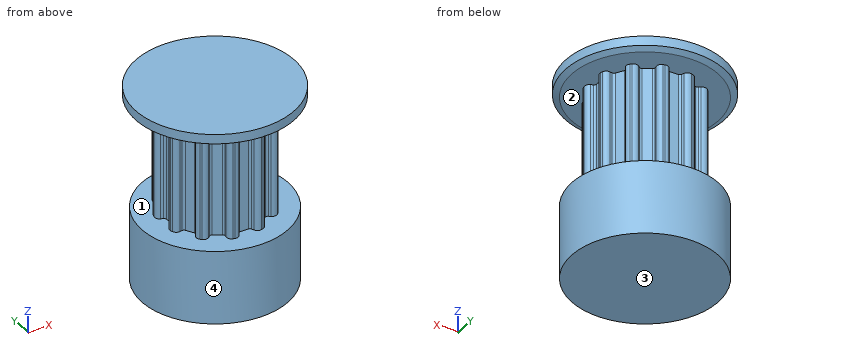
```python
from build123d import *

# Parameters (mm, degrees)
SKETCH5_W           = 10
SKETCH5_H           = 4.5
SKETCH16_W          = 6
SKETCH16_H          = 6
CUT_TOOTH_DEPTH     = 10
PATTERN_TOOTH_COUNT = 12


with BuildPart() as part:
    # Sketch5 → body (revolve)
    with BuildSketch(Plane(origin=(0, 0, 0), x_dir=(0, 0, -1), z_dir=(1, 0, 0))):
        with Locations((5, 2.25)):
            Rectangle(SKETCH5_W, SKETCH5_H)
    revolve(axis=Axis((0, 0, 0), (0, 0, -1)))

    # Sketch16 → body-hub (revolve)
    with BuildSketch(Plane(origin=(0, 0, 0), x_dir=(0, 0, -1), z_dir=(1, 0, 0))):
        with Locations((13, 3)):
            Rectangle(SKETCH16_W, SKETCH16_H)
    revolve(axis=Axis((0, 0, -16), (0, 0, 1)))

    # Sketch23 → cut-tooth (cut)
    with BuildSketch(Plane.XY):
        with BuildLine():
            Line((0.547897017, 3.931595971), (0.6147699, 4.11532771))
            ThreePointArc((0.6147699, 4.11532771), (0.802803604, 4.331669589), (1.087295431, 4.366667911))
            Line((1.087295431, 4.366667911), (1.087295431, 4.933335822))
            Line((1.087295431, 4.933335822), (-1.087295431, 4.933335822))
            Line((-1.087295431, 4.933335822), (-1.087295431, 4.366667911))
            ThreePointArc((-1.087295431, 4.366667911), (-0.802803604, 4.331669589), (-0.6147699, 4.11532771))
            Line((-0.6147699, 4.11532771), (-0.547897017, 3.931595971))
            ThreePointArc((-0.547897017, 3.931595971), (-0.47467378, 3.836169591), (-0.359958492, 3.8))
            Line((-0.359958492, 3.8), (0.359958492, 3.8))
            ThreePointArc((0.359958492, 3.8), (0.47467378, 3.836169591), (0.547897017, 3.931595971))
        make_face()
    cut_tooth = extrude(amount=-CUT_TOOTH_DEPTH, mode=Mode.SUBTRACT)

    # pattern-tooth: cut-tooth ×12 about axis
    pattern_tooth_axis = Axis((0, 0, -10), (0, 0, 1))
    for i in range(1, PATTERN_TOOTH_COUNT):
        add(cut_tooth.rotate(pattern_tooth_axis, i * 360 / PATTERN_TOOTH_COUNT), mode=Mode.SUBTRACT)

    # Sketch25 → body-flange-front (revolve)
    with BuildSketch(Plane(origin=(0, 0, 0), x_dir=(0, 0, -1), z_dir=(1, 0, 0))):
        Polygon((1, 3.25), (0, 3.25), (0, 5.416666667), (0, 6.5), (1, 6.5), (1, 5.416666667), align=None)
    revolve(axis=Axis((0, 0, 0), (0, 0, -1)))

    # Sketch28 → body-flange-profile-front (revolve, cut)
    with BuildSketch(Plane(origin=(0, 0, 0), x_dir=(0, 0, -1), z_dir=(1, 0, 0))):
        Polygon((1, 6.5), (1, 6), (0.766846171, 6.5), align=None)
    revolve(axis=Axis((0, 0, -10), (0, 0, 1)), mode=Mode.SUBTRACT)


solid = part.part
```
Part model, mm, in its own coordinate system. Face numbers are marked on the shaded views. Give positions to 0.01 mm unless a question says otherwise; leave off trailing zeros. Write each loop counter-clockwise with the first axis right and the second up, starting at its lowest first coordinate (ties: lowest second). Pieces come first, ordered by that corner, then holes. Notation, with made-up numbers: M 69,6 L 92,6 A34 cw 92,44 Z; hole C -30,80 d7. An arc over 180 degrees is marked long. Use CSV: the item, a comma, the result in double quotes.
Item 1: Pull direction Z, two halves, no side cores. Call the marked faces 1, 2, 3 and 4: +Z half, -Z half, draft (parallel to the pull), parting line (faces both ways), or undercut.
Taken from the geometry:
face 1,"undercut"
face 2,"undercut"
face 3,"-Z half"
face 4,"draft"
Item 2: Slice it at A-A on y = 0. Write the cut outline in (x, z), plus the area to 3 significant figures.
Taken from the geometry:
outline,"M -6.5,-0.77 L -6,-1 L -3.8,-1 L -3.8,-10 L -6,-10 L -6,-16 L 6,-16 L 6,-10 L 3.8,-10 L 3.8,-1 L 6,-1 L 6.5,-0.77 L 6.5,0 L -6.5,0 Z"
area,"153 mm²"
Item 3: Pin check, flat tips, straight feed: P1, Ø2, axis at y = 2, z = -6, coming from the -X side; P2, Ø0.6, axis at y = 0, z = -6, coming from the +X side; P3, Ø3, axis at y = -2.5, z = -13, coming from the +X side. Stop position of each tip, or through.
Taken from the geometry:
P1,"stops at x = -4.38"
P2,"stops at x = 3.8"
P3,"stops at x = 5.92"
Item 4: Drill centre lines: probe 1 along Z at (x, y) = (-3, 5); probe 2 along Y at (x, z) = (0, -12.5); probe 3 along Y at (x, z) = (-1, -6.5). Where is each one in solid material? Low to high.
Taken from the geometry:
probe 1,"z = -16 to -10, -1 to 0"
probe 2,"y = -6 to 6"
probe 3,"y = -4.38 to 4.38"
Item 5: Slice it at C-C on z = -11.25. Write the cut outline in (x, y).
Taken from the geometry:
outline,"C 0,0 d12"
